Check sheet for the modelled part. Datum: model origin and axes. Units: mm. Coordinates: 2 decimals unless noted, no trailing zeros. Loops run counter-clockwise (first coordinate to the right, second up) from the corner with the lowest first, then second, coordinate; pieces in that order, holes last. Notation, with made-up numbers: M 22,44.25 L 69,44.25 A12 cw 69,59.25 Z; hole C -27.5,88.5 d8. An arc over 180 degrees is marked long. Write each question's results on one line, items separated by ' | '. Start each with the question number.
from build123d import *

# Parameters (mm, degrees)
SKETCH1_W           = 370
SKETCH1_H           = 26.131621187
BOSS_EXTRUDE1_DEPTH = 2
SKETCH2_R           = 9
CUT_EXTRUDE1_DEPTH  = 2
SKETCH2_4_R         = 9
CUT_EXTRUDE2_DEPTH  = 2


with BuildPart() as part:
    # Sketch1 → Boss-Extrude1 (new body)
    with BuildSketch(Plane.XY):
        with Locations((60.280898876, 7.126805778)):
            Rectangle(SKETCH1_W, SKETCH1_H)
    extrude(amount=BOSS_EXTRUDE1_DEPTH)

    # Sketch2 → Cut-Extrude1 (cut)
    with BuildSketch(Plane.XY.offset(2)):
        with Locations((-109.719101124, 7.126805778)):
            Circle(SKETCH2_R)
    extrude(amount=-CUT_EXTRUDE1_DEPTH, mode=Mode.SUBTRACT)

    # Sketch2<4> → Cut-Extrude2 (cut)
    with BuildSketch(Plane.XY.offset(2)):
        with Locations((-109.719101124, 7.126805778)):
            Circle(SKETCH2_4_R)
        with Locations((230.280898876, 7.126805778)):
            Circle(SKETCH2_4_R)
    extrude(amount=-CUT_EXTRUDE2_DEPTH, mode=Mode.SUBTRACT)


solid = part.part
Item 1: Depth check by flat-ended pin: P1, Ø14.5, axis at x = -109.72, y = 7.13, coming from the +Z side. Enter the tip coordinate at first touch or a pass-through.
Item 2: Section check A-A (y = 2.25). Record the cut outline in (x, z), plus the area to 3 significant figures.
Item 3: Section check B-B (z = 1.1). Record the cut outline in (x, y), plus the area to 3 significant figures.
Item 4: Release check for a two-part mould opening along Y. For faces 1 (the face through (58, 7, 2)), 2 (the face through (238.865, 9.83, 1.014)) record: +Y half, -Y half, draft (parallel to the pull), parting line (faces both ways), or undercut.
Item 5: Thickness scan on line 1 (X direction, y = 8, z = 1.75); line 2 (X direction, y = 6, z = 0.4). Record the ranges inside material, lowest first.
Computed values:
1) P1: passes through
2) outline: M -124.72,0 L -117.28,0 L -117.28,2 L -124.72,2 Z; M -102.15,0 L 222.72,0 L 222.72,2 L -102.15,2 Z; M 237.85,0 L 245.28,0 L 245.28,2 L 237.85,2 Z | area: 679 mm²
3) outline: M -124.72,-5.94 L 245.28,-5.94 L 245.28,20.19 L -124.72,20.19 Z; hole C -109.72,7.13 d18; hole C 230.28,7.13 d18 | area: 9,160 mm²
4) face 1: draft | face 2: undercut
5) line 1: x = -124.72 to -118.68, -100.76 to 221.32, 239.24 to 245.28 | line 2: x = -124.72 to -118.65, -100.79 to 221.35, 239.21 to 245.28
